Can you work these out from the model? Positions are in its coordinate system, mm. A direction names the side the tool comes from. Give positions to 0.01 mm unless a question says otherwise; leave off trailing zeros. Loops run counter-clockwise (first coordinate to the right, second up) from the corner with the lowest first, then second, coordinate; pieces in that order, holes last.
from build123d import *

# Parameters (mm, degrees)
F0_R     = 3.75
F1_DEPTH = 17.5
F3_DEPTH = 25
F4_R     = 2.5


with BuildPart() as f1:
    # F0 (on Top) → F1 (new body)
    with BuildSketch(Plane.XY):
        with BuildLine():
            ThreePointArc((-40.66784, 7.5), (-45.971141, -5.303301), (-33.16784, 0))
            ThreePointArc((-33.16784, 0), (-35.364539, 5.303301), (-40.66784, 7.5))
        make_face()
        with Locations((-40.66784, 0)):
            Circle(F0_R, mode=Mode.SUBTRACT)
        with BuildLine():
            ThreePointArc((-40.66784, 7.5), (-35.364539, 5.303301), (-33.16784, 0))
            Line((-33.16784, 0), (-5.66784, 0))
            Line((-5.66784, 0), (-5.66784, 7.5))
            Line((-5.66784, 7.5), (-40.66784, 7.5))
        make_face()
    extrude(amount=F1_DEPTH)

    # F2 (on face) → F3 (cut)
    with BuildSketch(Plane.XZ):
        with BuildLine():
            Line((-5.66784, 5.625), (-5.66784, 11.875))
            Line((-5.66784, 11.875), (-25.66784, 11.875))
            ThreePointArc((-25.66784, 11.875), (-28.79284, 8.75), (-25.66784, 5.625))
            Line((-25.66784, 5.625), (-5.66784, 5.625))
        make_face()
    extrude(amount=-F3_DEPTH, mode=Mode.SUBTRACT)

    # F4
    f4_edges = [f1.edges().sort_by_distance(p)[0] for p in [
        (-5.66784, 3.75, 17.5),
        (-5.66784, 3.75, 0),
        (-33.16784, 0, 8.75),
    ]]
    fillet(f4_edges, radius=F4_R)


solid = f1.part
(1) Please list where these lines run through material, in increasing order: probe 1 along Z at (x, y) = (-11, 2.5) (3 decimals); probe 2 along Y at (x, z) = (-11, 1.75); probe 3 along Z at (x, y) = (-26.5, 2).
Returned:
probe 1: z = 0 to 5.625, 11.875 to 17.5
probe 2: y = 0 to 7.5
probe 3: z = 0 to 5.74, 11.76 to 17.5
(2) Will these pins go through, and if not, where does the flat tip stop? P1, Ø9, axis at x = -19.5, z = 10.5, coming from the -Y side; P2, Ø2, axis at x = -34.5, z = 4, coming from the -Y side; P3, Ø6, axis at x = -40.67, y = 0, coming from the +Z side.
Returned:
P1: stops at y = 0
P2: stops at y = -5.44
P3: passes through
(3) Suppose I cut it at A-A on x = -22. List the corners of the cut face in (y, z) for me (3 decimals).
Returned:
outline: (0, 0) - (7.5, 0) - (7.5, 5.625) - (0, 5.625) - close; (0, 11.875) - (7.5, 11.875) - (7.5, 17.5) - (0, 17.5) - close
(4) Suppose I cut it at D-D on y = 6. List the corners of the cut face in (x, z) for me (3 decimals).
Returned:
outline: (-45.168, 0) - (-8.168, 0) arc R2.5 ccw to (-5.668, 2.5) - (-5.668, 5.625) - (-25.668, 5.625) arc R3.125 cw to (-25.668, 11.875) - (-5.668, 11.875) - (-5.668, 15) arc R2.5 ccw to (-8.168, 17.5) - (-45.168, 17.5) - close
(5) Suppose I cut it at B-B on y = 2.75. List the corners of the cut face in (x, z) for me (3 decimals).
Returned:
outline: (-47.645, 0) - (-43.217, 0) - (-43.217, 17.5) - (-47.645, 17.5) - close; (-38.118, 0) - (-8.168, 0) arc R2.5 ccw to (-5.668, 2.5) - (-5.668, 5.625) - (-25.668, 5.625) arc R3.125 cw to (-25.668, 11.875) - (-5.668, 11.875) - (-5.668, 15) arc R2.5 ccw to (-8.168, 17.5) - (-38.118, 17.5) - close
(6) Which directions (+Z, -Z, +X, -X, +Y, -Y) give clear straight access to the entire face, cutting with the end or side of a thin tool? Please do faces 4 (the cylindrical face through (-6.42, 3.8, 16.79)), 5 (the flat face through (-19, 0, 5)), 6 (the flat face through (-16, 4, 5.625)).
Returned:
face 4: +Z, +X, +Y, -Y
face 5: +Z, -Z, +X, -Y
face 6: +X, +Y, -Y
(7) Thinking about a two-plate mould opening in X: for faces 1 (the flat face through (-28, 2, 17.5)), 2 (the flat face through (-5.668, 4, 13)), 3 (the cylindrical face through (-44.414, 0.165, 8.628)), which applies, pulls with the +X half, pulls with the -X half, needs draft (parallel to the pull), parting line crosses it, or undercut?
Returned:
face 1: needs draft
face 2: pulls with the +X half
face 3: undercut
(8) Suppose I cut it at C-C on z = 14.25. List the corners of the cut face in (x, y) for me (3 decimals), plus the area to 3 significant figures.
Returned:
outline: (-40.668, 7.5) arc R7.5 ccw (long way) to (-33.406, -1.875) arc R2.5 cw to (-30.985, 0) - (-5.668, 0) - (-5.668, 7.5) - close; hole circle Ø7.5 at (-40.668, 0)
area: 352 mm2
